```python
from build123d import *

# Parameters (mm, degrees)
F0_W         = 8
F0_H         = 8
F1_DEPTH     = 2.5
F2_R         = 3
F3_R         = 2
F4_DEPTH     = 90
F5_W         = 8
F5_H         = 2
F6_DEPTH     = 25
F7_T4_DEPTH  = 32.7638593636
F7_S5_R      = 2
F7_T6_DEPTH  = 19
F7_T10_DEPTH = 32.7638593636
F7_S11_R     = 2
F7_T12_DEPTH = 19


# Not quite as in the source:
# - a fillet or chamfer that OpenCascade refuses, or shapes differently, is made with other operations: its cross-section is extruded or revolved along the edge and cut away or added


with BuildPart() as f1:
    # F0 (on Top) → F1 (new body)
    with BuildSketch(Plane.XY):
        with Locations((-11.3665966003, 7.8844996169)):
            Rectangle(F0_W, F0_H)
    extrude(amount=F1_DEPTH)

    # F2
    f2_edges = [f1.edges().sort_by_distance(p)[0] for p in [
        (-15.366597, 3.8845, 1.25),
        (-15.366597, 11.8845, 1.25),
        (-7.366597, 3.8845, 1.25),
        (-7.366597, 11.8845, 1.25),
    ]]
    fillet(f2_edges, radius=F2_R)

    # F3 (on face) → F4 (join)
    with BuildSketch(Plane.XY.offset(2.5)):
        with Locations((-11.3665966003, 7.8844996169)):
            Circle(F3_R)
    extrude(amount=F4_DEPTH)

    # F5 (on face) → F6 (join)
    with BuildSketch(Plane.XY.offset(2.5)):
        with Locations((-11.3665966003, 7.8844996169)):
            Rectangle(F5_W, F5_H)
    extrude(amount=F6_DEPTH)

    # F7: chamfer of 5 on 2 edges, made by hand


with BuildPart() as f7_tool2:
    # F7_s3 → F7_t4 (new body)
    with BuildSketch(Plane.XZ.offset(-24.2664292987)):
        with BuildLine():
            Line((-16.427256772, 21.4393398282), (-9.3059364285, 28.5606601718))
            Line((-9.3059364285, 28.5606601718), (-9.3059364285, 29.3106601718))
            ThreePointArc((-9.3059364285, 29.3106601718), (-12.3362665144, 28.25), (-15.3665966003, 28.25))
            Line((-15.3665966003, 28.25), (-16.1165966003, 27.5))
            ThreePointArc((-16.1165966003, 27.5), (-16.1165966003, 24.4696699141), (-17.177256772, 21.4393398282))
            Line((-17.177256772, 21.4393398282), (-16.427256772, 21.4393398282))
        make_face()
    extrude(amount=F7_T4_DEPTH)

    # F7_s5 → F7_t6 (cut, symmetric)
    with BuildSketch(Plane.XY.offset(25.4)):
        with Locations((-11.3665966003, 7.8844996169)):
            Circle(F7_S5_R)
    extrude(amount=F7_T6_DEPTH, both=True, mode=Mode.SUBTRACT)


with BuildPart() as f1_1:
    add(f1.part)

    # F7_t1: cut F7_tool2
    add(f7_tool2.part, mode=Mode.SUBTRACT)


with BuildPart() as f7_tool8:
    # F7_s9 → F7_t10 (new body)
    with BuildSketch(Plane.XZ.offset(8.4974300649)):
        with BuildLine():
            Line((-6.3059364285, 21.4393398282), (-13.427256772, 28.5606601718))
            Line((-13.427256772, 28.5606601718), (-13.427256772, 29.3106601718))
            ThreePointArc((-13.427256772, 29.3106601718), (-10.3969266861, 28.25), (-7.3665966003, 28.25))
            Line((-7.3665966003, 28.25), (-6.6165966003, 27.5))
            ThreePointArc((-6.6165966003, 27.5), (-6.6165966003, 24.4696699141), (-5.5559364285, 21.4393398282))
            Line((-5.5559364285, 21.4393398282), (-6.3059364285, 21.4393398282))
        make_face()
    extrude(amount=-F7_T10_DEPTH)

    # F7_s11 → F7_t12 (cut, symmetric)
    with BuildSketch(Plane.XY.offset(25.4)):
        with Locations((-11.3665966003, 7.8844996169)):
            Circle(F7_S11_R)
    extrude(amount=F7_T12_DEPTH, both=True, mode=Mode.SUBTRACT)


with BuildPart() as f1_2:
    add(f1_1.part)

    # F7_t7: cut F7_tool8
    add(f7_tool8.part, mode=Mode.SUBTRACT)


solid = f1_2.part
```
Could you check a few things on this model? Use its own coordinates, in mm. A direction names the side the tool comes from. Coordinates: 2 decimals unless noted, no trailing zeros. Loops run counter-clockwise (first coordinate to the right, second up) from the corner with the lowest first, then second, coordinate; pieces in that order, holes last. Notation, with made-up numbers: M -11,88 L 38,88 A36 ccw 38,124 Z; hole C 33.25,57.5 d7. An arc over 180 degrees is marked long. Put each result on its own line as item: value. Start each with the question number.
(1) Suppose I cut it at A-A on z = 13. Please give me the cut outline in (x, y).
(2) Suppose I cut it at B-B on y = 5. Please give me the cut outline in (x, z).
(3) I need wall thicknesses on line 1 (Z direction, x = -9.25, y = 9.5); line 2 (Y direction, x = -15, z = 13.5); line 3 (X direction, y = 9.5, z = 14). Which ranges of each line are inside material? Lowest first, please. Write a range as from..to.
(4) Will these pins go through, and if not, where does the flat tip stop? P1, Ø2, axis at x = -10, z = 13.5, coming from the +Y side; P2, Ø3, axis at y = 10, z = 26, coming from the -X side; P3, Ø2.5, axis at x = -14.5, z = 17.5, coming from the -Y side; P4, Ø1.5, axis at x = -11, y = 5.5, coming from the +Z side.
(5) Suppose I cut it at C-C on z = 35. Please give me the cut outline in (x, y), then the cut area to 3 significant figures.
(6) For faces 1 (the face through (-9, 8.884, 13)), 2 (the face through (-11, 5, 2.5)), 3 (the face through (-14, 6.884, 13)), which set-ups out of +Z, -Z, +X, -X, +Y, -Y let a thin tool reach every point of the face, with its end or its side?
Solutions:
1. outline: M -15.37,6.88 L -13.1,6.88 A2 ccw -9.63,6.88 L -7.37,6.88 L -7.37,8.88 L -9.63,8.88 A2 ccw -13.1,8.88 L -15.37,8.88 Z
2. outline: M -14.7,0 L -8.03,0 L -8.03,2.5 L -14.7,2.5 Z
3. line 1: z = 0..2.5
3. line 2: y = 6.88..8.88
3. line 3: x = -12.55..-10.19
4. P1: stops at y = 9.85
4. P2: stops at x = -13.27
4. P3: stops at y = 6.88
4. P4: stops at z = 92.5
5. outline: C -11.37,7.88 d4
5. area: 12.6 mm2
6. face 1: +Z, +X, +Y
6. face 2: +Z, -Y
6. face 3: +Z, -X, -Y
